Check sheet for the drawn part. Datum: minimum x, y, z corner. Units: mm. Coordinates: 2 decimals unless noted, no trailing zeros. Write each loop counter-clockwise with the first axis right and the second up, starting at its lowest first coordinate (ties: lowest second). Pieces come first, ordered by that corner, then holes. Notation, with made-up numbers: (35.5, 32.25) -> (53.5, 32.25) arc R18 cw to (53.5, 63.25) -> close; hole circle Ø6 at (5, 21.5). An arc over 180 degrees is marked (long way). Write item = value, one per line. Start each with the question number.
(1) Section check B-B (y = 6). Record the cut outline in (x, z) (1 decimal), plus the area to 3 significant figures.
(2) Section check A-A (x = 110). Record the cut outline in (y, z).
(3) Section check D-D (x = 36.5). Record the cut outline in (y, z).
(4) Material ranges on probe 1 along Z at (x, y) = (108, 2) (1 decimal); probe 2 along Z at (x, y) = (93, 6) (1 decimal); probe 3 along Z at (x, y) = (59.5, 2.5), recorded low to high. Write a range as [from, to].
(5) Section check C-C (z = 83). Record the cut outline in (x, y).
(6) Gauge pin test, flat ends, axial feed: pin 1 Ø3 at (y, z) = (3, 22) entering from +X; pin 2 Ø1 at (x, y) = (121, 7) entering from +Z; pin 3 Ø1.5 at (y, z) = (7, 32.5) entering from -X. Record the tip position at first contact, or that the pin passes through.
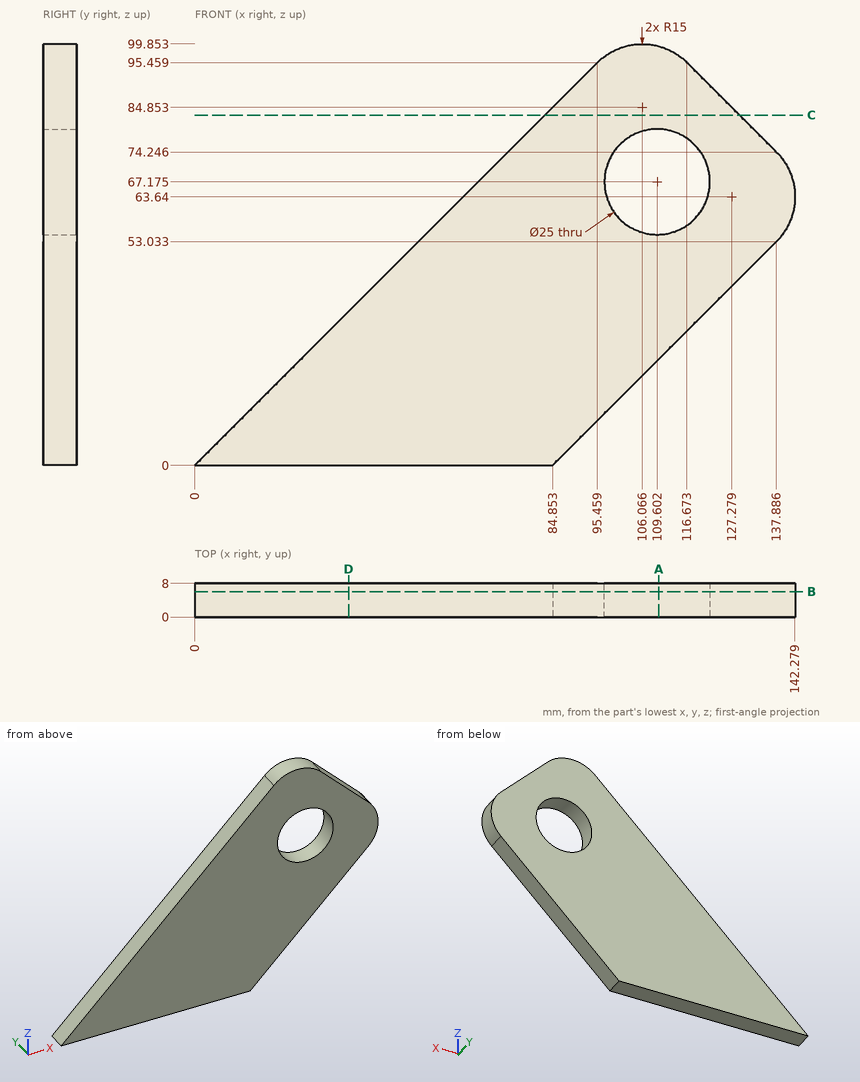
Response:
q1.outline = (0, 0) -> (84.9, 0) -> (137.9, 53) arc R15 ccw to (137.9, 74.2) -> (116.7, 95.5) arc R15 ccw to (95.5, 95.5) -> close; hole circle Ø25 at (109.6, 67.2)
q1.area = 6,610 mm2
q2.outline = (0, 25.15) -> (8, 25.15) -> (8, 54.68) -> (0, 54.68) -> close; (0, 79.67) -> (8, 79.67) -> (8, 99.33) -> (0, 99.33) -> close
q3.outline = (0, 0) -> (8, 0) -> (8, 36.5) -> (0, 36.5) -> close
q4.probe_1 = [23.1, 54.8], [79.6, 99.7]
q4.probe_2 = [8.1, 93]
q4.probe_3 = [0, 59.5]
q5.outline = (83, 0) -> (129.13, 0) -> (129.13, 8) -> (83, 8) -> close
q6.pin_1 = 108.35
q6.pin_2 = 91.63
q6.pin_3 = 31.75
